Print and shaded views of the part. All mm, measured from the part's lowest x, y and z. Coordinates: 2 decimals unless noted, no trailing zeros. Loops run counter-clockwise (first coordinate to the right, second up) from the corner with the lowest first, then second, coordinate; pieces in that order, holes last. Notation, with made-up numbers: M 5,57 L 17,57 A10 ccw 17,67 Z; hole C 70.25,9.5 d11. An arc over 180 degrees is marked long. One line per question, with ' | ' between items. Start each with the question number.
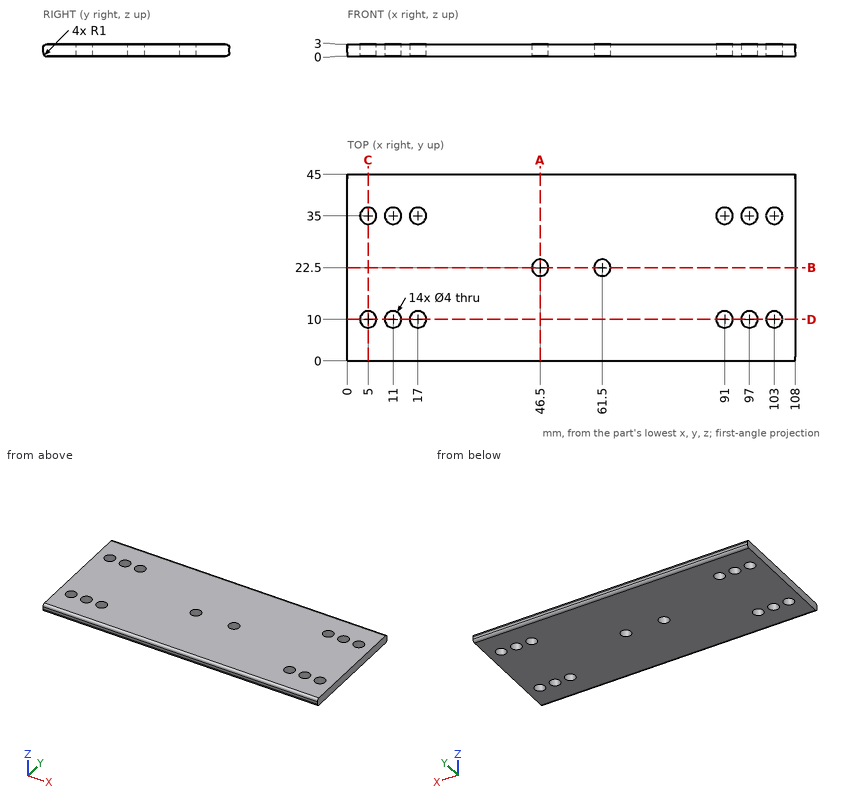
(1) Drill centre lines: line 1 (Y direction, x = 61.5, z = 0.95); line 2 (Y direction, x = 103, z = 0.9); line 3 (Y direction, x = 11, z = 2.35). Where is each one in solid material? Low to high. Write a range as [from, to].
(2) Band-saw the part on C-C on x = 5. Write the cut outline in (y, z), then the cut area to 3 significant figures.
(3) Pin check, flat tip, straight feed: P1, Ø2.5, axis at x = 103, y = 10, coming from the +Z side. Stop position of the tip, or through.
(4) Band-saw the part on A-A on x = 46.5. Write the cut outline in (y, z).
(5) Band-saw the part on D-D on y = 10. Write the cut outline in (x, z).
(6) Band-saw the part on B-B on y = 22.5. Write the cut outline in (x, z), then the cut area to 3 significant figures.
Computed values:
1) line 1: [0, 20.5], [24.5, 45] | line 2: [0.01, 8], [12, 33], [37, 44.99] | line 3: [0.06, 8], [12, 33], [37, 44.94]
2) outline: M 0,1 A1 ccw 1,0 L 8,0 L 8,3 L 1,3 A1 ccw 0,2 Z; M 12,0 L 33,0 L 33,3 L 12,3 Z; M 37,0 L 44,0 A1 ccw 45,1 L 45,2 A1 ccw 44,3 L 37,3 Z | area: 110 mm^2
3) P1: through
4) outline: M 0,1 A1 ccw 1,0 L 20.5,0 L 20.5,3 L 1,3 A1 ccw 0,2 Z; M 24.5,0 L 44,0 A1 ccw 45,1 L 45,2 A1 ccw 44,3 L 24.5,3 Z
5) outline: M 0,0 L 3,0 L 3,3 L 0,3 Z; M 7,0 L 9,0 L 9,3 L 7,3 Z; M 13,0 L 15,0 L 15,3 L 13,3 Z; M 19,0 L 89,0 L 89,3 L 19,3 Z; M 93,0 L 95,0 L 95,3 L 93,3 Z; M 99,0 L 101,0 L 101,3 L 99,3 Z; M 105,0 L 108,0 L 108,3 L 105,3 Z
6) outline: M 0,0 L 44.5,0 L 44.5,3 L 0,3 Z; M 48.5,0 L 59.5,0 L 59.5,3 L 48.5,3 Z; M 63.5,0 L 108,0 L 108,3 L 63.5,3 Z | area: 300 mm^2
